For this review, use the dimensioned drawing (mm, ordinates from the lowest corner) and the shaded views. Round coordinates to 2 decimals unless told otherwise and drop trailing zeros. Loops run counter-clockwise (first coordinate to the right, second up) from the corner with the lowest first, then second, coordinate; pieces in that order, holes last. Notation, with made-up numbers: (59.5, 64.25) -> (94.5, 64.25) arc R19 ccw to (94.5, 70.25) -> close; hole circle Ø10 at (-0.5, 41.25). An arc over 180 degrees is marked (long way). Write each question's results on one line, items separated by ' | '. Start each with the question number.
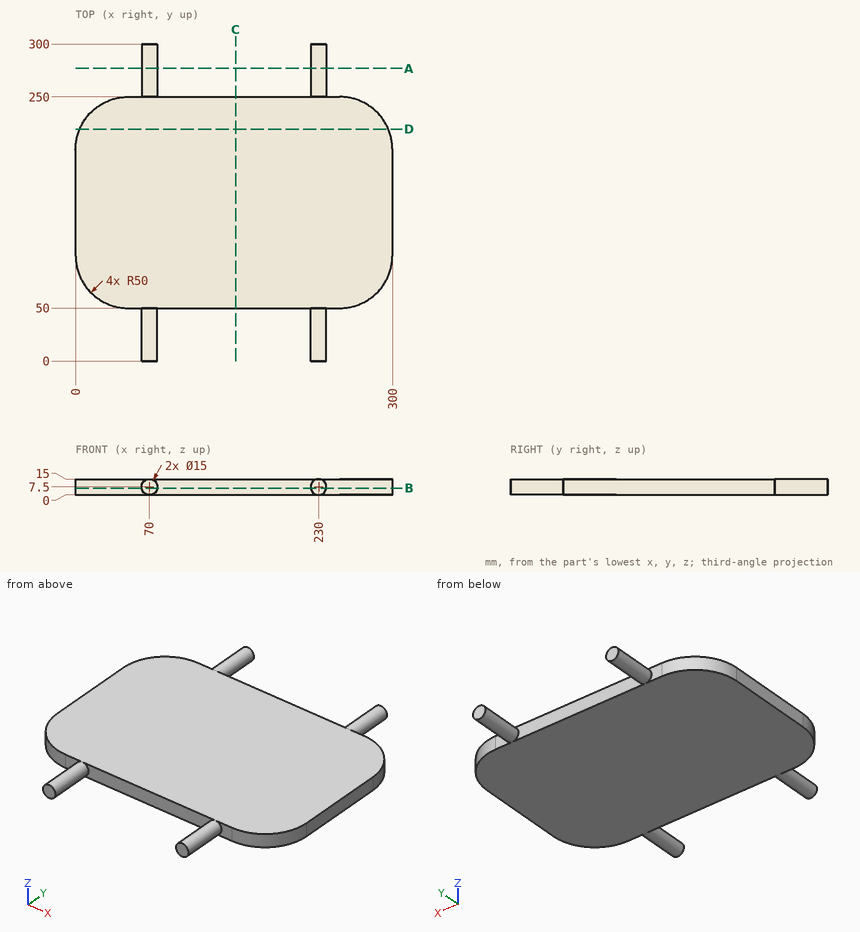
1) Take a section at C-C (x = 151.5). Write out the cut boundary in (y, z), plus the area to 3 significant figures.
2) Take a section at B-B (z = 6.25). Write out the cut boundary in (x, y), plus the area to 3 significant figures.
3) To check wall thickness, follow line 1 (Y direction, x = 81, z = 3.5); line 2 (X direction, y = 267, z = 7); line 3 (X direction, y = 201.5, z = 2.75). State the ranges of each line that lie inside material, in increasing order. Write a range as from..to.
4) Take a section at D-D (y = 219.5). Write out the cut boundary in (x, z), plus the area to 3 significant figures.
5) Take a section at A-A (y = 277). Write out the cut boundary in (x, z).
6) Insertion check: pin 1 (4.5 mm diameter, centred on x = 134, z = 9.5, fed in from +Y); pin 2 (4.5 mm diameter, centred on x = 131, z = 5.5, fed in from -Y). Each pin has a flat end and moves straight along its axis. Give the tip position at first contact, or say it passes through.
Geometry check:
1) outline: (50, 0) -> (250, 0) -> (250, 15) -> (50, 15) -> close | area: 3,000 mm^2
2) outline: (0, 100) arc R50 ccw to (50, 50) -> (62.6, 50) -> (62.6, 0) -> (77.4, 0) -> (77.4, 50) -> (222.6, 50) -> (222.6, 0) -> (237.4, 0) -> (237.4, 50) -> (250, 50) arc R50 ccw to (300, 100) -> (300, 200) arc R50 ccw to (250, 250) -> (237.4, 250) -> (237.4, 300) -> (222.6, 300) -> (222.6, 250) -> (77.4, 250) -> (77.4, 300) -> (62.6, 300) -> (62.6, 250) -> (50, 250) arc R50 ccw to (0, 200) -> close | area: 60,800 mm^2
3) line 1: y = 50..250 | line 2: x = 62.52..77.48, 222.52..237.48 | line 3: x = 0.02..299.98
4) outline: (3.96, 0) -> (296.04, 0) -> (296.04, 15) -> (3.96, 15) -> close | area: 4,380 mm^2
5) outline: circle Ø15 at (70, 7.5); circle Ø15 at (230, 7.5)
6) pin 1: stops at y = 250 | pin 2: stops at y = 50
